For this review, take the finished solid that the model builds, in its own axes (mm). Coordinates: 2 decimals unless noted, no trailing zeros. Loops run counter-clockwise (first coordinate to the right, second up) from the corner with the lowest first, then second, coordinate; pieces in that order, holes last. Notation, with made-up numbers: (5, 77) -> (11, 77) arc R27 cw to (11, 93) -> close; hole circle Ø6 at (-35, 30.25). An arc over 180 degrees is marked (long way). Use a Markdown table: item, result.
from build123d import *

# Parameters (mm, degrees)
SKETCH1_W                = 12
SKETCH1_H                = 109.262
BOSS_EXTRUDE1_DEPTH      = 4
FILLET1_R                = 5
CUT_EXTRUDE1_DEPTH       = 10.5
SKETCH4_W                = 12
SKETCH4_H                = 6.738165359
BOSS_EXTRUDE2_DEPTH      = 4
BOSS_EXTRUDE3_DEPTH      = 6
BOSS_EXTRUDE3_DEPTH_BACK = 4
SKETCH5_W                = 14
SKETCH5_H                = 122.000165359
SKETCH6_R                = 3.25
CUT_EXTRUDE3_DEPTH       = 10
FILLET2_R                = 5
LPATTERN1_COUNT          = 7
LPATTERN1_PITCH          = 18


with BuildPart() as part:
    # Sketch1 → Boss-Extrude1 (new body)
    with BuildSketch(Plane.XY):
        with Locations((0, 50)):
            Rectangle(SKETCH1_W, SKETCH1_H)
    extrude(amount=BOSS_EXTRUDE1_DEPTH)

    # Fillet1
    fillet1_edges = [part.edges().sort_by_distance(p)[0] for p in [
        (-6, -4.631, 2),
        (6, -4.631, 2),
    ]]
    fillet(fillet1_edges, radius=FILLET1_R)

    # Sketch2 → Cut-Extrude1 (cut)
    with BuildSketch(Plane.XY.offset(4)):
        with BuildLine():
            Line((2, 98.631), (2, 1.369))
            ThreePointArc((2, 1.369), (0, -0.631), (-2, 1.369))
            Line((-2, 1.369), (-2, 98.631))
            ThreePointArc((-2, 98.631), (0, 100.631), (2, 98.631))
        make_face()
    extrude(amount=-CUT_EXTRUDE1_DEPTH, mode=Mode.SUBTRACT)

    # Sketch4 → Boss-Extrude2 (add)
    with BuildSketch(Plane.XY.offset(4)):
        with Locations((0, 108.000082679)):
            Rectangle(SKETCH4_W, SKETCH4_H)
    extrude(amount=-BOSS_EXTRUDE2_DEPTH)

    # Sketch5 → Boss-Extrude3 (add, two sides: drawn at the far end of the back side and taken through both)
    with BuildSketch(Plane(origin=(0, 0, 0), x_dir=(-1, 0, 0), z_dir=(0, 0, -1)).offset(-BOSS_EXTRUDE3_DEPTH_BACK)):
        with Locations((0, 56.36908268)):
            Rectangle(SKETCH5_W, SKETCH5_H)
    extrude(amount=BOSS_EXTRUDE3_DEPTH + BOSS_EXTRUDE3_DEPTH_BACK)

    # Sketch6 → Cut-Extrude3 (cut)
    with BuildSketch(Plane(origin=(0, 0, -6), x_dir=(-1, 0, 0), z_dir=(0, 0, -1))):
        with Locations((0, 110.369165359)):
            Circle(SKETCH6_R)
    cut_extrude3 = extrude(amount=-CUT_EXTRUDE3_DEPTH, mode=Mode.SUBTRACT)

    # Fillet2
    fillet2_edges = [part.edges().sort_by_distance(p)[0] for p in [
        (-7, -4.631, -1),
        (-7, 117.369165359, -1),
        (7, 117.369165359, -1),
        (7, -4.631, -1),
    ]]
    fillet(fillet2_edges, radius=FILLET2_R)

    # LPattern1: Cut-Extrude3 ×7
    with Locations(*[(0, -i * LPATTERN1_PITCH, 0) for i in range(1, LPATTERN1_COUNT)]):
        add(cut_extrude3, mode=Mode.SUBTRACT)


solid = part.part
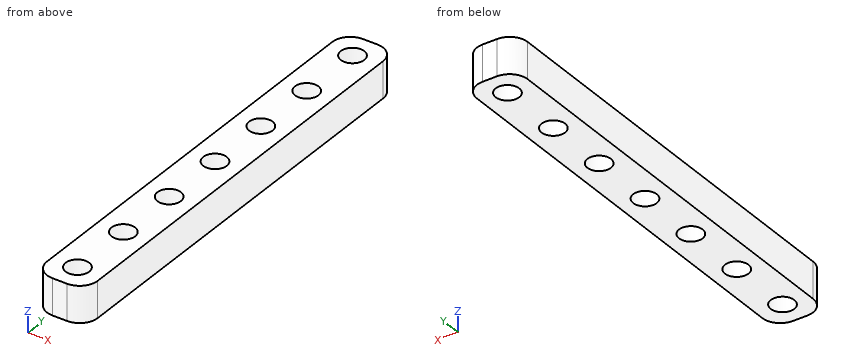
(1) Take a section at B-B on z = -3.25. Write out the cut boundary in (x, y), plus the area to 3 significant figures.
Found:
| item | result |
|---|---|
| outline | (-7, 0.37) arc R5 ccw to (-2, -4.63) -> (2, -4.63) arc R5 ccw to (7, 0.37) -> (7, 112.37) arc R5 ccw to (2, 117.37) -> (-2, 117.37) arc R5 ccw to (-7, 112.37) -> close; hole circle Ø6.5 at (0, 2.37); hole circle Ø6.5 at (0, 20.37); hole circle Ø6.5 at (0, 38.37); hole circle Ø6.5 at (0, 56.37); hole circle Ø6.5 at (0, 74.37); hole circle Ø6.5 at (0, 92.37); hole circle Ø6.5 at (0, 110.37) |
| area | 1,450 mm^2 |
(2) Take a section at A-A on x = 0. State how many separate pieces and enclosed holes the cut face has, plus the area to 3 significant figures.
Found:
| item | result |
|---|---|
| separate pieces | 8 |
| enclosed holes | 0 |
| area | 765 mm^2 |
(3) For pin 1 Ø2 at (x, z) = (-4, -2.5) entering from -Y, flat-tipped, find the tip position at first contact; note if it passes through.
Found:
| item | result |
|---|---|
| pin 1 | stops at y = -4.53 |
(4) For line 1 along X through (y, z) = (94, 1.75); line 2 along X through (y, z) = (21, -4); line 3 along Y through (x, z) = (3.5, -3.25), list the stretches that pass through material, from the lowest coordinate up.
Found:
| item | result |
|---|---|
| line 1 | x = -7 to -2.81, 2.81 to 7 |
| line 2 | x = -7 to -3.19, 3.19 to 7 |
| line 3 | y = -4.4 to 117.14 |
